```python
from build123d import *

# Parameters (mm, degrees)
F1_DEPTH  = 63.5
F3_DEPTH  = 63.5
F4_W      = 228.6
F4_H      = 16.6908878535
F6_DEPTH  = 82.55
F12_DEPTH = 63.5


with BuildPart() as f1:
    # F0 (on Front) → F1 (new body)
    with BuildSketch(Plane.XZ):
        Polygon((-31.75, -219.075), (22.225, -219.075), (31.75, 136.525), (31.75, 219.075), (-31.75, 219.075), align=None)
    extrude(amount=F1_DEPTH)

    # F2 (on face) → F3 (cut)
    with BuildSketch(Plane(origin=(-31.75, 0, 0), x_dir=(0, -1, 0), z_dir=(-1, 0, 0))):
        Polygon((9.525, -219.075), (0, 136.525), (0, -219.075), align=None)
    extrude(amount=-F3_DEPTH, mode=Mode.SUBTRACT)

    # F5: F1 across plane


with BuildPart() as f1_1:
    add(f1.part)
    add(f1.part.mirror(Plane.YZ))

    # F4 (on face) → F6 (join)
    with BuildSketch(Plane.XY.offset(219.075)):
        with Locations((146.05, -39.2795560732)):
            Rectangle(F4_W, F4_H)
    extrude(amount=-F6_DEPTH)

    # F11 (on face) → F12 (cut)
    with BuildSketch(Plane.XZ.offset(63.5)):
        Polygon((31.75, -219.075), (31.75, 136.525), (22.225, -219.075), align=None)
    extrude(amount=-F12_DEPTH, mode=Mode.SUBTRACT)

    # F13: F1 across plane


with BuildPart() as f1_2:
    add(f1_1.part)
    add(f1_1.part.mirror(Plane(origin=(146.05, -47.625, 219.075), x_dir=(0, 1, 0), z_dir=(1, 0, 0))))


solid = f1_2.part
```
Part model, mm, in its own coordinate system. A direction names the side the tool comes from. Round coordinates to 2 decimals unless told otherwise and drop trailing zeros. Write each loop counter-clockwise with the first axis right and the second up, starting at its lowest first coordinate (ties: lowest second). Pieces come first, ordered by that corner, then holes.
Item 1: Which spindle directions (+Z, -Z, +X, -X, +Y, -Y) get a long thin tool onto all of the face, cutting with end or side? Do faces 4 (the flat face through (143.6, -31.3, 219.075)), 5 (the flat face through (260.35, -15, 178)), 6 (the flat face through (144, -39, 136.525)), 7 (the flat face through (144, -47.625, 178)), 8 (the flat face through (-31.75, -31, 3)). Say none if no direction does.
Results:
face 4: +Z, +X, -X, +Y, -Y
face 5: +Z, -Z, +Y
face 6: -Z, +Y, -Y
face 7: +Z, -Z, -Y
face 8: +Z, -Z, -X, +Y, -Y
Item 2: Cut at A-A, the plane y = -19.5. Give the cut face in (x, z) (3 decimals).
Results:
outline: (-31.75, -219.075) - (22.225, -219.075) - (31.75, 136.525) - (31.75, 219.075) - (-31.75, 219.075) - close; (260.35, 136.525) - (269.875, -219.075) - (323.85, -219.075) - (323.85, 219.075) - (260.35, 219.075) - close
Item 3: Cut at C-C, the plane y = -39.5. Give the cut face in (x, z) (3 decimals).
Results:
outline: (-31.75, -219.075) - (22.225, -219.075) - (31.75, 136.525) - (260.35, 136.525) - (269.875, -219.075) - (323.85, -219.075) - (323.85, 219.075) - (-31.75, 219.075) - close
Item 4: Probe L1, parallel to Z at x = 231.5, y = -38 (3 decimals); L2, parallel to X at y = -21, z = 153.5; L3, parallel to X at y = -50, z = 117. List the from-to ranges inside material, lowest first.
Results:
L1: z = 136.525 to 219.075
L2: x = -31.75 to 31.75, 260.35 to 323.85
L3: x = -31.75 to 31.23, 260.87 to 323.85
Item 5: Cut at D-D, the plane x = -5.5. Give the cut face in (y, z) (3 decimals), plus the area to 3 significant figures.
Results:
outline: (-63.5, -219.075) - (-9.525, -219.075) - (0, 136.525) - (0, 219.075) - (-63.5, 219.075) - close
area: 26,100 mm2
Item 6: Cut at B-B, the plane z = -19. Give the cut face in (x, y), plus the area to 3 significant figures.
Results:
outline: (-31.75, -63.5) - (27.58, -63.5) - (27.58, -4.17) - (-31.75, -4.17) - close; (264.52, -63.5) - (323.85, -63.5) - (323.85, -4.17) - (264.52, -4.17) - close
area: 7,040 mm2
Item 7: Drop a flat-ended pin along its axis: pin 1 Ø8.5 at (x, y) = (171, -39.5) entering from -Z (3 decimals). Give the stop position or say it passes through.
Results:
pin 1: stops at z = 136.525
Item 8: Two-plate mould, pull along X, no slides. Class faces 1 (the flat face through (260.35, -55, 178)), 2 (the flat face through (323.85, -31, 3)), 3 (the flat face through (292, -63.5, 3)): +X half, -X half, draft (parallel to the pull), parting line (faces both ways), or undercut.
Results:
face 1: undercut
face 2: +X half
face 3: draft
